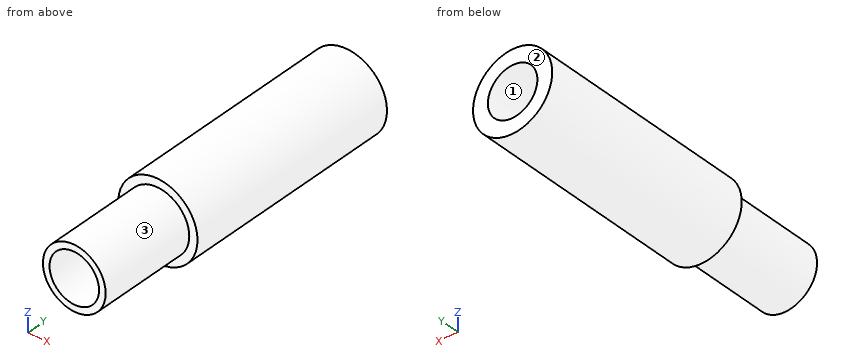
Autodesk Fusion 360 part; units mm, degrees
sketch "Sketch1" plane through (0, 0, 0) normal (0, 1, 0) x (1, 0, 0)
  circle A0 centre (0, 0) radius 12
  circle A1 centre (0, 0) radius 7.5
  circle A2 centre (0, 0) radius 9.5
extrude "Extrude1" add sketch "Sketch1" along normal blind 45 contours A0 | A2
extrude "Extrude2" add sketch "Sketch1" against normal blind 25 contours A2
extrude "Extrude3" add sketch "Sketch1" against normal blind 11 contours A0
extrude "Extrude4" add 1 faces at (8.77, -25, 0.8446) along direction (0, -1, 0) blind 16
extrude "Extrude5" add 1 faces at (11.0866, -11, 1.0681) along direction (0, -1, 0) blind 14
extrude "Extrude6" add 1 faces at (8.77, -41, 0.8446) along direction (0, -1, 0) blind 14
extrude "Extrude8" cut 1 faces at (10.4274, 45, 0.9688) along direction (0, -1, 0) blind 2
extrude "Extrude7" [suppressed]
Verification items for the finished model (mm, model axes). Face numbers are marked on the shaded views. Give positions to 0.01 mm unless a question says otherwise; leave off trailing zeros. Order: outer loops, then holes, each group sorted by start corner. A loop starts at its lowest first (then second) coordinate and runs counter-clockwise, first axis right, second up. Notation, with made-up numbers: M -24.5,80 L 21.5,80 A29 cw 21.5,113 Z; hole C -20.75,-20 d7. An arc over 180 degrees is marked long. Use one line per item in the form item = value. Start each with the question number.
Q1. Go/stop test with flat-tipped pins: pin 1 Ø5 at (x, y) = (-8.5, 14.5) entering from +Z; pin 2 Ø4 at (y, z) = (-30, 6) entering from +X; pin 3 Ø6 at (x, y) = (7, -22.5) entering from +Z. Record where each tip stops, or that it passes through.
Q2. Section check A-A (z = 0). Enter the section's corners in (x, y), then the cut area to 3 significant figures.
Q3. Scan lines: line 1 along Z through (x, y) = (0, -27.5); line 2 along Z through (x, y) = (0, 23.5). Record each from-to range of solid material in increasing order. Write a range as [from, to].
Q4. Mould release check, pull along Z, two halves, no side actions. Record for the marked faces 1, 2 and 3: +Z half, -Z half, draft (parallel to the pull), parting line (faces both ways), or undercut.
Q5. Section check B-B (x = 0). Enter the section's corners in (y, z), then the cut area to 3 significant figures.
Q6. Section check C-C (y = 34). Enter the section's corners in (x, z).
Evaluation:
q1.pin_1 = 10.39
q1.pin_2 = 8.62
q1.pin_3 = 11.31
q2.outline = M -12,-25 L -9.5,-25 L -9.5,-55 L -7.5,-55 L -7.5,43 L -12,43 Z; M 7.5,-55 L 9.5,-55 L 9.5,-25 L 12,-25 L 12,43 L 7.5,43 Z
q2.area = 732 mm2
q3.line_1 = [-9.5, -7.5], [7.5, 9.5]
q3.line_2 = [-12, -7.5], [7.5, 12]
q4.face_1 = undercut
q4.face_2 = draft
q4.face_3 = parting line
q5.outline = M -55,-9.5 L -25,-9.5 L -25,-12 L 43,-12 L 43,-7.5 L -55,-7.5 Z; M -55,7.5 L 43,7.5 L 43,12 L -25,12 L -25,9.5 L -55,9.5 Z
q5.area = 732 mm2
q6.outline = C 0,0 d24; hole C 0,0 d15
